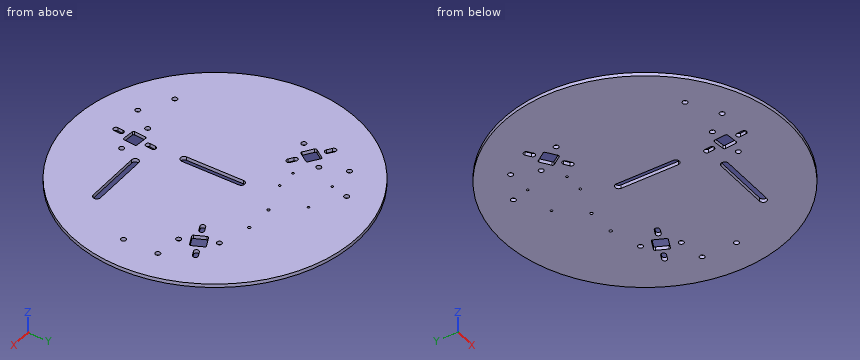
from build123d import *

# Parameters (mm, degrees)
SKETCH1_R           = 200
BOSS_EXTRUDE2_DEPTH = 5
SKETCH9_R           = 3.5
CUT_EXTRUDE8_DEPTH  = 5
CIRPATTERN5_COUNT   = 3
SKETCH15_R          = 2
CUT_EXTRUDE13_DEPTH = 5
SKETCH17_R          = 3.5
CUT_EXTRUDE15_DEPTH = 5
CIRPATTERN7_COUNT   = 3
CUT_EXTRUDE16_DEPTH = 5
CUT_EXTRUDE17_DEPTH = 5
SKETCH20_R          = 1.6
CUT_EXTRUDE18_DEPTH = 5
FILLET1_R           = 2


with BuildPart() as part:
    # Sketch1 → Boss-Extrude2 (new body)
    with BuildSketch(Plane.XY):
        Circle(SKETCH1_R)
    extrude(amount=BOSS_EXTRUDE2_DEPTH)

    # Sketch9 → Cut-Extrude8 (cut)
    with BuildSketch(Plane.XY.offset(5)):
        with Locations((-56.715390309, 146.233937587)):
            Circle(SKETCH9_R)
        with Locations((-98.284609691, 122.233937587)):
            Circle(SKETCH9_R)
    cut_extrude8 = extrude(amount=-CUT_EXTRUDE8_DEPTH, mode=Mode.SUBTRACT)

    # CirPattern5: Cut-Extrude8 ×3 about axis
    cirpattern5_axis = Axis((0, 0, 0), (0, 0, 1))
    for i in range(1, CIRPATTERN5_COUNT):
        add(cut_extrude8.rotate(cirpattern5_axis, i * 360 / CIRPATTERN5_COUNT), mode=Mode.SUBTRACT)

    # Sketch15 → Cut-Extrude13 (cut)
    with BuildSketch(Plane.XY.offset(5)):
        with Locations((15, 85)):
            Circle(SKETCH15_R)
        with Locations((55, 85)):
            Circle(SKETCH15_R)
    extrude(amount=-CUT_EXTRUDE13_DEPTH, mode=Mode.SUBTRACT)

    # Sketch17 → Cut-Extrude15 (cut)
    with BuildSketch(Plane.XY.offset(5)):
        with Locations((-84.532410842, 88.488821425)):
            Circle(SKETCH17_R)
        with Locations((-112.064079787, 49.169523299)):
            Circle(SKETCH17_R)
        Polygon((-112.225530121, 66.373416283), (-95.842489235, 54.901887556), (-84.370960508, 71.284928442), (-100.754001394, 82.756457169), align=None)
        with BuildLine():
            Line((-79.907686902, 60.22467579), (-73.354470547, 55.636064299))
            ThreePointArc((-73.354470547, 55.636064299), (-72.49495592, 50.761514617), (-77.369505602, 49.901999989))
            Line((-77.369505602, 49.901999989), (-83.922721956, 54.49061148))
            ThreePointArc((-83.922721956, 54.49061148), (-84.782236584, 59.365161162), (-79.907686902, 60.22467579))
        make_face()
        with BuildLine():
            Line((-112.673768673, 83.167733244), (-119.226985028, 87.756344735))
            ThreePointArc((-119.226985028, 87.756344735), (-124.10153471, 86.896830107), (-123.242020082, 82.022280425))
            Line((-123.242020082, 82.022280425), (-116.688803728, 77.433668934))
            ThreePointArc((-116.688803728, 77.433668934), (-111.814254045, 78.293183562), (-112.673768673, 83.167733244))
        make_face()
    cut_extrude15 = extrude(amount=-CUT_EXTRUDE15_DEPTH, mode=Mode.SUBTRACT)

    # CirPattern7: Cut-Extrude15 ×3 about axis
    cirpattern7_axis = Axis((0, 0, 0), (0, 0, 1))
    for i in range(1, CIRPATTERN7_COUNT):
        add(cut_extrude15.rotate(cirpattern7_axis, i * 360 / CIRPATTERN7_COUNT), mode=Mode.SUBTRACT)

    # Sketch18 → Cut-Extrude16 (cut)
    with BuildSketch(Plane.XY.offset(5)):
        with BuildLine():
            Line((-5, 30), (-5, -50))
            ThreePointArc((-5, -50), (-10, -55), (-15, -50))
            Line((-15, -50), (-15, 30))
            ThreePointArc((-15, 30), (-10, 35), (-5, 30))
        make_face()
    extrude(amount=-CUT_EXTRUDE16_DEPTH, mode=Mode.SUBTRACT)

    # Sketch19 → Cut-Extrude17 (cut)
    with BuildSketch(Plane.XY.offset(5)):
        with BuildLine():
            Line((25, -90), (105, -90))
            ThreePointArc((105, -90), (110, -95), (105, -100))
            Line((105, -100), (25, -100))
            ThreePointArc((25, -100), (20, -95), (25, -90))
        make_face()
    extrude(amount=-CUT_EXTRUDE17_DEPTH, mode=Mode.SUBTRACT)

    # Sketch20 → Cut-Extrude18 (cut)
    with BuildSketch(Plane.XY.offset(5)):
        with Locations((-63, 121.9)):
            Circle(SKETCH20_R)
        with Locations((-15, 120.8)):
            Circle(SKETCH20_R)
        with Locations((-58.3, 70)):
            Circle(SKETCH20_R)
        with Locations((-30.4, 70)):
            Circle(SKETCH20_R)
    extrude(amount=-CUT_EXTRUDE18_DEPTH, mode=Mode.SUBTRACT)

    # Fillet1
    fillet1_edges = [part.edges().sort_by_distance(p)[0] for p in [
        (-1.368299576, -130.376868179, 2.5),
        (-21.292193538, -128.633753324, 2.5),
        (-19.549078683, -108.709859363, 2.5),
        (0.374815279, -110.452974218, 2.5),
        (113.593829697, 64.003451897, 2.5),
        (122.046194932, 45.877296156, 2.5),
        (103.920039191, 37.424930921, 2.5),
        (95.467673957, 55.551086662, 2.5),
        (-112.225530121, 66.373416283, 2.5),
        (-100.754001394, 82.756457169, 2.5),
        (-84.370960508, 71.284928442, 2.5),
        (-95.842489235, 54.901887556, 2.5),
    ]]
    fillet(fillet1_edges, radius=FILLET1_R)


solid = part.part
Source: CAD feature listing. Evaluate the final solid. Frame: model axes, mm. Round coordinates to 2 decimals unless told otherwise and drop trailing zeros. Loops run counter-clockwise (first coordinate to the right, second up) from the corner with the lowest first, then second, coordinate; pieces in that order, holes last. Notation, with made-up numbers: (85, 59) -> (124, 59) arc R28 cw to (124, 83) -> close; hole circle Ø2 at (20.5, 79). An arc over 180 degrees is marked (long way). Answer as a JSON object with one key per item and string values. Group by question number.
Q1. Contact query for flat-ended pins moving along their axis: P1, Ø3, axis at x = 122, z = 2.5, coming from the -Y side; P2, Ø3, axis at x = -134, z = 4, coming from the +Y side; P3, Ø2, axis at x = -42.5, z = 1, coming from the -Y side. Output: stop coordinate, or through.
Q2. Section query A-A (y = 0). Output: boundary loops of the cut face in (x, z), plus the area to 3 significant figures.
Q3. Section query C-C (z = 2.15). State how many separate pieces and enclosed holes the cut face has, plus the area to 3 significant figures.
Q4. Section query B-B (x = 37.5). Output: boundary loops of the cut face in (y, z), plus the area to 3 significant figures.
Q5. Section query D-D (y = 160.5). Output: boundary loops of the cut face in (x, z), plus the area to 3 significant figures.
Q6. Ray query, line 1 (X direction, y = 122.5, z = 1.75); line 2 (X direction, y = 75.5, z = 3.35); line 3 (X direction, y = 120.8, z = 2.2). Return the intervals inside material, ascending. Write a range as from..to.
Completed:
{
 "1": {"P1": "y = -159.62", "P2": "y = 149.81", "P3": "y = -195.65"},
 "2": {"outline": "(-200, 0) -> (-15, 0) -> (-15, 5) -> (-200, 5) -> close; (-5, 0) -> (200, 0) -> (200, 5) -> (-5, 5) -> close", "area": "1,950 mm²"},
 "3": {"separate pieces": "1", "enclosed holes": "29", "area": "122,000 mm²"},
 "4": {"outline": "(-196.45, 0) -> (-100, 0) -> (-100, 5) -> (-196.45, 5) -> close; (-90, 0) -> (196.45, 0) -> (196.45, 5) -> (-90, 5) -> close", "area": "1,910 mm²"},
 "5": {"outline": "(-119.33, 0) -> (119.33, 0) -> (119.33, 5) -> (-119.33, 5) -> close", "area": "1,190 mm²"},
 "6": {"line 1": "-158.09..-101.77, -94.79..-64.48, -61.52..158.09", "line 2": "-185.2..-105.84, -90.39..96.87, 100.36..185.2", "line 3": "-159.4..-101.48, -95.09..-64.16, -61.84..-16.6, -13.4..159.4"}
}
